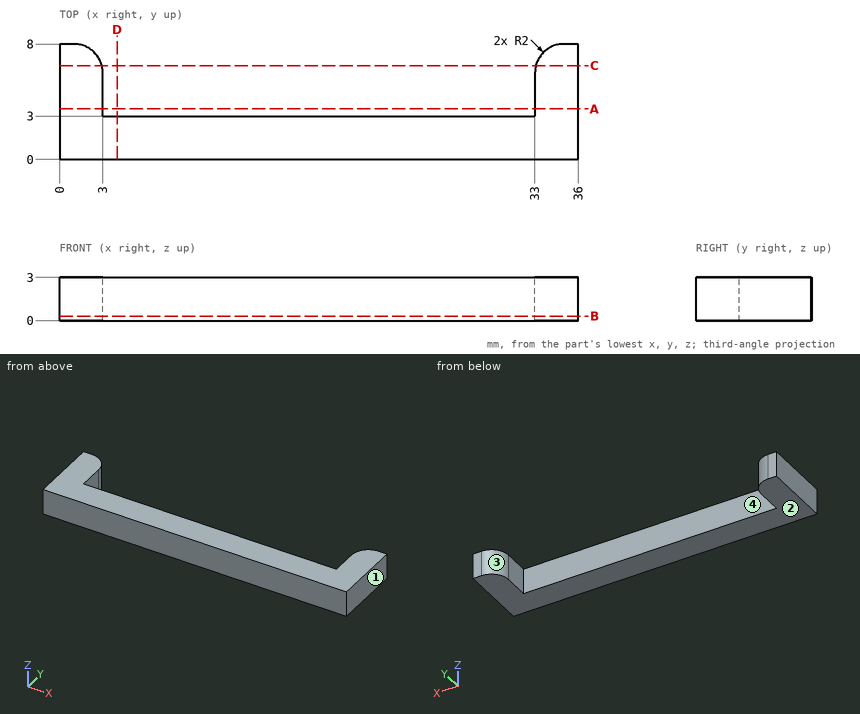
Job drawing, mm, ordinate dimensions from the low corner. One solid piece. Give positions to 0.01 mm unless a question says otherwise; leave off trailing zeros. Loops run counter-clockwise (first coordinate to the right, second up) from the corner with the lowest first, then second, coordinate; pieces in that order, holes last. Notation, with made-up numbers: (30, 19) -> (81, 19) arc R19 cw to (81, 38) -> close; hole circle Ø9 at (59.25, -29). An arc over 180 degrees is marked (long way). Write each question's results on one line, items separated by ' | '. Start each with the question number.
Q1. Band-saw the part on A-A on y = 3.5. List the corners of the cut face in (x, z).
Q2. Band-saw the part on B-B on z = 0.3. List the corners of the cut face in (x, y).
Q3. Wall check: L1, parallel to X at y = 3.25, z = 0.8; L2, parallel to Y at x = 11, z = 1.95; L3, parallel to X at y = 6.5, z = 2.1. Give the ranges that are in metal, low to high.
Q4. Band-saw the part on D-D on x = 4. List the corners of the cut face in (y, z), plus the area to 3 significant figures.
Q5. Pin check, flat tip, straight feed: P1, Ø1.5, axis at x = 25.5, z = 1.5, coming from the +Y side. Stop position of the tip, or through.
Q6. Band-saw the part on C-C on y = 6.5. List the corners of the cut face in (x, z).
Q7. Pull direction X, two halves, no side cores. Call the marked faces 1, 2, 3 and 4: +X half, -X half, draft (parallel to the pull), parting line (faces both ways), or undercut.
Results are:
1) outline: (0, 0) -> (3, 0) -> (3, 3) -> (0, 3) -> close; (33, 0) -> (36, 0) -> (36, 3) -> (33, 3) -> close
2) outline: (0, 0) -> (36, 0) -> (36, 8) -> (35, 8) arc R2 ccw to (33, 6) -> (33, 3) -> (3, 3) -> (3, 6) arc R2 ccw to (1, 8) -> (0, 8) -> close
3) L1: x = 0 to 3, 33 to 36 | L2: y = 0 to 3 | L3: x = 0 to 2.94, 33.06 to 36
4) outline: (0, 0) -> (3, 0) -> (3, 3) -> (0, 3) -> close | area: 9.00 mm²
5) P1: stops at y = 3
6) outline: (0, 0) -> (2.94, 0) -> (2.94, 3) -> (0, 3) -> close; (33.06, 0) -> (36, 0) -> (36, 3) -> (33.06, 3) -> close
7) face 1: +X half | face 2: draft | face 3: undercut | face 4: undercut
